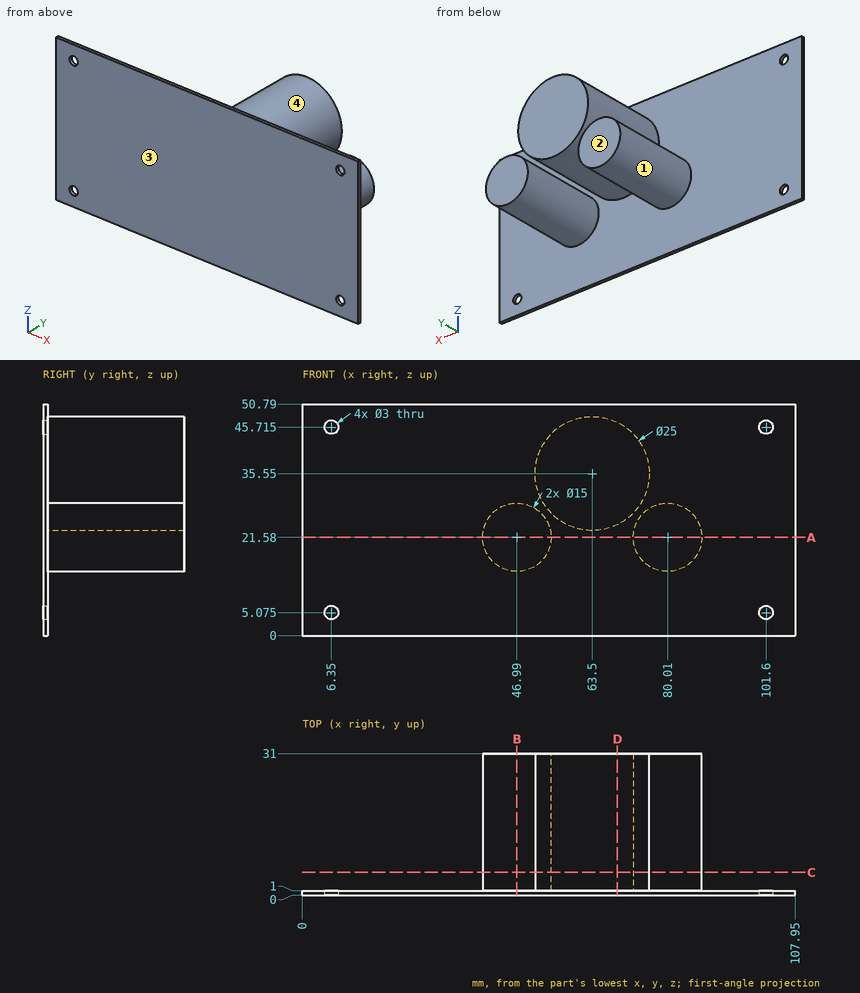
Could you check a few things on this drawing? It's one solid part, dimensions in mm from its lowest x, y, z. A direction names the side the tool comes from. Coordinates: 2 decimals unless noted, no trailing zeros. Loops run counter-clockwise (first coordinate to the right, second up) from the corner with the lowest first, then second, coordinate; pieces in that order, holes last. Notation, with made-up numbers: (22, 3.5) - (47, 3.5) arc R31 ccw to (47, 42.5) - close; hole circle Ø2 at (-5, 8). An arc over 180 degrees is marked (long way). Answer as a JSON object with one key per item and string values. Group by question number.
Item 1: If we section it at B-B (x = 46.99): List the corners of the cut face in (y, z) for me.
Item 2: On a 3-axis mill with a long thin cutter (end or side, diameter ignored), from which of +Z, -Z, +X, -X, +Y, -Y can I reach the whole of each face in a straight line? I mean the marked faces 1 and 2. Say none if no direction works.
Item 3: If we section it at D-D (x = 69): List the corners of the cut face in (y, z) for me.
Item 4: For pin 1 (3 mm diameter, centred on y = 19, z = 37.5, fed in from +X); pin 2 (12 mm diameter, centred on y = 14, z = 10.5, fed in from +X); pin 3 (3.5 mm diameter, centred on x = 101.6, z = 5.075, fed in from +Y), each with a flat end and sliding along its axis, tell me the tip position at first contact or that it passes through.
Item 5: If we section it at A-A (z = 21.58): List the corners of the cut face in (x, y) for me.
Item 6: If we mould it in two halves opening along Z, with no side actions, what happens to the marked faces 3 and 4? For each: released by +Z, released by -Z, zero draft, split by the parting line, or undercut.
Item 7: If I drill on L1, parallel to Z at x = 6.35, y = 0.8 (3 decimals); L2, parallel to X at y = 14, z = 25; L3, parallel to X at y = 18, z = 35.5, over which ranges is the centre line in solid material (lowest first)? Write a range as from..to.
Item 8: If we section it at C-C (y = 5): List the corners of the cut face in (x, z) for me.
Returned:
{
 "1": {"outline": "(0, 0) - (1, 0) - (1, 14.08) - (31, 14.08) - (31, 29.08) - (1, 29.08) - (1, 50.79) - (0, 50.79) - close"},
 "2": {"face 1": "+Y", "face 2": "+Z, -Z, +X, -X, +Y"},
 "3": {"outline": "(0, 0) - (1, 0) - (1, 24.33) - (31, 24.33) - (31, 46.77) - (1, 46.77) - (1, 50.79) - (0, 50.79) - close"},
 "4": {"pin 1": "stops at x = 75.99", "pin 2": "stops at x = 85.53", "pin 3": "stops at y = 1"},
 "5": {"outline": "(0, 0) - (107.95, 0) - (107.95, 1) - (87.51, 1) - (87.51, 31) - (72.51, 31) - (72.51, 1) - (54.49, 1) - (54.49, 31) - (39.49, 31) - (39.49, 1) - (0, 1) - close"},
 "6": {"face 3": "zero draft", "face 4": "undercut"},
 "7": {"L1": "z = 0..3.575, 6.575..44.215, 47.215..50.79", "L2": "x = 40.32..53.66, 56.8..70.2, 73.34..86.68", "L3": "x = 51..76"},
 "8": {"outline": "circle Ø15 at (46.99, 21.58); circle Ø25 at (63.5, 35.55); circle Ø15 at (80.01, 21.58)"}
}
